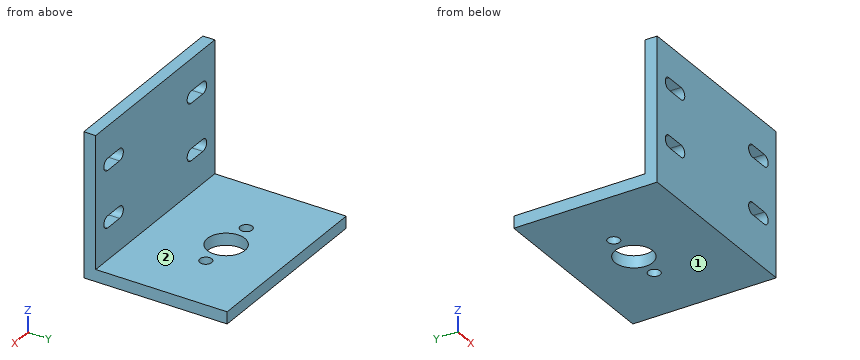
Autodesk Inventor part; units mm, degrees
ref_plane "YZ Plane" through (0, 0, 0) normal (1, 0, 0) x (0, 1, 0)
ref_plane "XZ Plane" through (0, 0, 0) normal (0, 1, 0) x (-1, 0, 0)
ref_plane "XY Plane" through (0, 0, 0) normal (0, 0, 1) x (1, 0, 0)
sketch "Sketch1" plane through (0, 0, 0) normal (0, 0, 1) x (1, 0, 0)
  line L0 (25, 16.8) -> (25, -19.8)
  line L1 (25, -19.8) -> (-25, -19.8)
  line L2 (-25, -19.8) -> (-25, 16.8)
  line L3 (-25, -19.8) -> (-25, -16.8)
  line L4 (-25, -19.8) -> (-25, 18.3)
  line L5 (-25, 18.3) -> (25, 18.3)
  line L6 (25, 18.3) -> (25, -19.8)
  line L7 (-25, -19.8) -> (-25, -16.625)
  line L8 (-25, -16.625) -> (25, -16.625)
  dimension "d94" = 3.175
extrude "Extrusion3" add sketch "Sketch1" along normal blind 3.175
extrude "Extrusion4" add sketch "Sketch1" along normal blind 38.1 contours L0 L1 L2 L8
sketch "Sketch2" plane through (-25, -16.625, 3) normal (0, 1, 0) x (1, 0, 0)
  line L0 (50, -35.1) -> (0, -35.1)
  line L1 (0, 0) -> (50, 0)
  line L2 (0, 0) -> (0, -35.1)
  line L3 (50, 0) -> (50, -35.1)
  line L4 (50, -35.1) -> (45, -35.1)
  line L5 (0, -35.1) -> (0, -25.1)
  line L6 (0, 3) -> (0, -35.1)
  line L7 (45, -35.1) -> (45, -25.1)
  line L8 (45, -25.1) -> (5, -25.1)
  line L9 (5, -25.1) -> (5, -10.1)
  line L10 (5, -10.1) -> (45, -10.1)
  line L11 (45, -10.1) -> (45, -25.1)
  point P0 (40, -25.1)
  point P1 (40, -10)
  point P2 (10, -10)
  point P3 (10, -25.1)
  dimension "d83" = 5
  dimension "d84" = 10
  dimension "d85" = 40
  dimension "d86" = 15
sketch "Sketch3" plane through (0, 0, 0) normal (0, 0, -1) x (-1, 0, 0)
  line L0 (25, 18.3) -> (25, -0.75)
  line L1 (-25, -16.8) -> (-25, 18.3)
  line L2 (25, 18.3) -> (25, 2.3)
  line L3 (25, 18.3) -> (25, -19.8)
  line L4 (0, 2.2) -> (0.1, 2.2)
  point P0 (0, -0.75)
  dimension "d67" = 19.05
  dimension "d68" = 25
  dimension "d95" = 16
  dimension "d98" = 0.1
hole "Hole4" at (0, 2.2, 0) direction (0, 0, 1) diameter 10 end through all
sketch "Sketch4" plane through (0, 0, 0) normal (0, 0, -1) x (-1, 0, 0)
  circle A0 centre (-8.5, 2.2) radius 1.2295
  circle A1 centre (8.5, 2.2) radius 1.2295
  line L0 (-25, 18.3) -> (25, 18.3)
  line L1 (25, 18.3) -> (25, 2.3)
  line L2 (25, 18.3) -> (25, -19.8)
  line L3 (8.5, 2.2) -> (-8.5, 2.1769)
  point P0 (0, 0)
  point P1 (8.5, 2.1769)
  dimension "d96" = 16
hole "Hole5" at (8.5, 2.1769, 0) at (-8.5, 2.1769, 0) direction (0, 0, 1) diameter 3.18 end through all
sketch "Sketch5" plane through (-25, -16.625, 3.175) normal (0, 1, 0) x (1, 0, 0)
  arc A0 (45, -26.515) -> (45, -23.335) centre (45, -24.925) ccw
  arc A1 (40, -23.335) -> (40, -26.515) centre (40, -24.925) ccw
  line L0 (45, -26.515) -> (40, -26.515)
  line L1 (40, -23.335) -> (45, -23.335)
  arc A2 (45, -11.515) -> (45, -8.335) centre (45, -9.925) ccw
  arc A3 (40, -8.335) -> (40, -11.515) centre (40, -9.925) ccw
  line L2 (45, -11.515) -> (40, -11.515)
  line L3 (40, -8.335) -> (45, -8.335)
  arc A4 (10, -26.515) -> (10, -23.335) centre (10, -24.925) ccw
  arc A5 (5, -23.335) -> (5, -26.515) centre (5, -24.925) ccw
  line L4 (10, -26.515) -> (5, -26.515)
  line L5 (5, -23.335) -> (10, -23.335)
  arc A6 (10, -11.515) -> (10, -8.335) centre (10, -9.925) ccw
  arc A7 (5, -8.335) -> (5, -11.515) centre (5, -9.925) ccw
  line L6 (10, -11.515) -> (5, -11.515)
  line L7 (5, -8.335) -> (10, -8.335)
  point P0 (25, 3.175)
extrude "Extrusion5" cut sketch "Sketch5" against normal blind 10
properties part number "Suportepara o motor em cantorneira"
Geometry: final body of the model. Coordinates: model frame, mm. Face numbers are marked on the shaded views. A direction names the side the tool comes from. Round coordinates to 2 decimals unless told otherwise and drop trailing zeros. Order: outer loops, then holes, each group sorted by start corner. A loop starts at its lowest first (then second) coordinate and runs counter-clockwise, first axis right, second up. Notation, with made-up numbers: (-22, -25.5) -> (-10, -25.5) arc R21 cw to (-10, 12.5) -> close; hole circle Ø3 at (-36, -20). An arc over 180 degrees is marked (long way). Use one line per item in the form item = value. Start each with the question number.
1. Cut plane B-B (z = 13.1). Return the cut outline in (x, y) (3 decimals).
2. Cut plane C-C (x = 18). Return the cut outline in (y, z) (3 decimals).
3. Reachability of the marked faces 1 and 2 from +Z, -Z, +X, -X, +Y, -Y: full face, straight path, thin tool, end or side. Return the list, or none.
4. Cut plane D-D (y = -2). Return the cut outline in (x, z) (3 decimals).
5. Line query: probe 1 along X at (y, z) = (2.2, 1.4); probe 2 along Y at (x, z) = (-8.5, 0.8); probe 3 along Y at (x, z) = (0, 1). Output: solid intervals per line, ascending.
6. Cut plane A-A (x = -4). Return the cut outline in (y, z) (3 decimals).
7. Pin query (flat end, axial travel): pin 1 Ø11.5 at (x, y) = (0, 2.2) entering from +Z (3 decimals); pin 2 Ø8 at (x, z) = (6.5, 28.5) entering from +Y (3 decimals). Return the tip coordinate at first contact, or that it passes through.
Solution:
q1.outline = (-25, -19.8) -> (-21.59, -19.8) -> (-21.59, -16.625) -> (-25, -16.625) -> close; (-13.41, -19.8) -> (13.41, -19.8) -> (13.41, -16.625) -> (-13.41, -16.625) -> close; (21.59, -19.8) -> (25, -19.8) -> (25, -16.625) -> (21.59, -16.625) -> close
q2.outline = (-19.8, 0) -> (18.3, 0) -> (18.3, 3.175) -> (-16.625, 3.175) -> (-16.625, 11.51) -> (-19.8, 11.51) -> close; (-19.8, 14.69) -> (-16.625, 14.69) -> (-16.625, 26.51) -> (-19.8, 26.51) -> close; (-19.8, 29.69) -> (-16.625, 29.69) -> (-16.625, 38.1) -> (-19.8, 38.1) -> close
q3.face_1 = -Z, +X, -X, +Y, -Y
q3.face_2 = +Z, +X, -X, +Y
q4.outline = (-25, 0) -> (-2.713, 0) -> (-2.713, 3.175) -> (-25, 3.175) -> close; (2.713, 0) -> (25, 0) -> (25, 3.175) -> (2.713, 3.175) -> close
q5.probe_1 = -25 to -10.09, -6.91 to -5, 5 to 6.91, 10.09 to 25
q5.probe_2 = -19.8 to 0.59, 3.77 to 18.3
q5.probe_3 = -19.8 to -2.8, 7.2 to 18.3
q6.outline = (-19.8, 0) -> (-0.8, 0) -> (-0.8, 3.175) -> (-16.625, 3.175) -> (-16.625, 38.1) -> (-19.8, 38.1) -> close; (5.2, 0) -> (18.3, 0) -> (18.3, 3.175) -> (5.2, 3.175) -> close
q7.pin_1 = 3.175
q7.pin_2 = -16.625
